Check sheet for the modelled part. Datum: model origin and axes. Units: mm. Face numbers are marked on the shaded views. Give positions to 0.01 mm unless a question says otherwise; leave off trailing zeros. Loops run counter-clockwise (first coordinate to the right, second up) from the corner with the lowest first, then second, coordinate; pieces in that order, holes last. Notation, with made-up numbers: M -23,-19.75 L 36,-19.75 A10 ccw 36,-9.75 Z; hole C 74,-27.5 d3. An arc over 180 degrees is marked long. Use one line per item in the form item = value.
from build123d import *

# Parameters (mm, degrees)
SKETCH_W      = 46.8
SKETCH_H      = 46.8
SKETCH_R      = 2.75
SKETCH_R_2    = 1.5
PAD_DEPTH     = 3
SKETCH001_R   = 5
SKETCH001_R_2 = 2.75
PAD001_DEPTH  = 4


with BuildPart() as part:
    # Sketch → Pad (new body)
    with BuildSketch(Plane.XY):
        with Locations((18.4, -18.4)):
            Rectangle(SKETCH_W, SKETCH_H)
        with Locations((10, -10)):
            Circle(SKETCH_R, mode=Mode.SUBTRACT)
        with Locations((30, -10)):
            Circle(SKETCH_R, mode=Mode.SUBTRACT)
        with Locations((30, -30)):
            Circle(SKETCH_R, mode=Mode.SUBTRACT)
        with Locations((10, -30)):
            Circle(SKETCH_R, mode=Mode.SUBTRACT)
        Circle(SKETCH_R_2, mode=Mode.SUBTRACT)
        with Locations((36.8, 0)):
            Circle(SKETCH_R_2, mode=Mode.SUBTRACT)
        with Locations((0, -36.8)):
            Circle(SKETCH_R_2, mode=Mode.SUBTRACT)
        with Locations((36.8, -36.8)):
            Circle(SKETCH_R_2, mode=Mode.SUBTRACT)
    extrude(amount=PAD_DEPTH)

    # Sketch001 → Pad001 (join)
    with BuildSketch(Plane.XY):
        with Locations((30, -10)):
            Circle(SKETCH001_R)
        with Locations((30, -10)):
            Circle(SKETCH001_R_2, mode=Mode.SUBTRACT)
        with Locations((10, -10)):
            Circle(SKETCH001_R)
        with Locations((10, -10)):
            Circle(SKETCH001_R_2, mode=Mode.SUBTRACT)
        with Locations((10, -30)):
            Circle(SKETCH001_R)
        with Locations((10, -30)):
            Circle(SKETCH001_R_2, mode=Mode.SUBTRACT)
        with Locations((30, -30)):
            Circle(SKETCH001_R)
        with Locations((30, -30)):
            Circle(SKETCH001_R_2, mode=Mode.SUBTRACT)
    extrude(amount=-PAD001_DEPTH)


solid = part.part
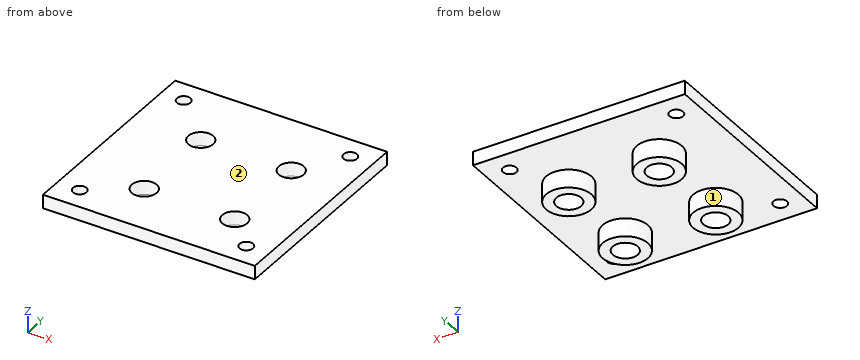
1) Section check B-B (y = -10). Record the cut outline in (x, z).
Evaluation:
outline = M -5,0 L 5,0 L 5,-4 L 7.25,-4 L 7.25,3 L -5,3 Z; M 12.75,-4 L 15,-4 L 15,0 L 25,0 L 25,-4 L 27.25,-4 L 27.25,3 L 12.75,3 Z; M 32.75,-4 L 35,-4 L 35,0 L 41.8,0 L 41.8,3 L 32.75,3 Z
2) Release check for a two-part mould opening along Y. For the marked faces 1 and 2 record: pulls with the +Y half, pulls with the -Y half, needs draft (parallel to the pull), parting line crosses it, or undercut.
Evaluation:
face_1 = undercut
face_2 = needs draft
3) Section check A-A (z = -2.5). Record the cut outline in (x, y), then the cut area to 3 significant figures.
Evaluation:
outline = C 10,-30 d10; C 10,-10 d10; C 30,-30 d10; C 30,-10 d10; hole C 10,-30 d5.5; hole C 10,-10 d5.5; hole C 30,-30 d5.5; hole C 30,-10 d5.5
area = 219 mm^2
4) Depth check by flat-ended pin: pin 1 Ø9 at (x, y) = (30, -30) entering from -Z; pin 2 Ø5 at (x, y) = (9, -1.5) entering from -Z; pin 3 Ø4.5 at (x, y) = (10, -10) entering from -Z. Enter the tip coordinate at first touch or a pass-through.
Evaluation:
pin_1 = -4
pin_2 = 0
pin_3 = through
5) Section check C-C (x = 10). Record the cut outline in (y, z), then the cut area to 3 significant figures.
Evaluation:
outline = M -41.8,0 L -35,0 L -35,-4 L -32.75,-4 L -32.75,3 L -41.8,3 Z; M -27.25,-4 L -25,-4 L -25,0 L -15,0 L -15,-4 L -12.75,-4 L -12.75,3 L -27.25,3 Z; M -7.25,-4 L -5,-4 L -5,0 L 5,0 L 5,3 L -7.25,3 Z
area = 143 mm^2
6) Scan lines: line 1 (Y direction, x = 30, z = -2); line 2 (Y direction, x = 10, z = 2.15); line 3 (Y direction, x = 0, z = 1.9). Record each from-to range of solid material in increasing order.
Evaluation:
line_1 = -35 to -32.75, -27.25 to -25, -15 to -12.75, -7.25 to -5
line_2 = -41.8 to -32.75, -27.25 to -12.75, -7.25 to 5
line_3 = -41.8 to -38.3, -35.3 to -1.5, 1.5 to 5
7) Section check D-D (z = 0.75). State how many separate pieces and enclosed holes the cut face has, then the cut area to 3 significant figures.
Evaluation:
separate_pieces = 1
enclosed_holes = 8
area = 2,070 mm^2
